Work out the finished part from the listing and answer in its coordinate system (mm). Give positions to 0.01 mm unless a question says otherwise; leave off trailing zeros. Loops run counter-clockwise (first coordinate to the right, second up) from the corner with the lowest first, then second, coordinate; pieces in that order, holes last. Notation, with made-up numbers: M 3,-31.75 L 56,-31.75 A25 cw 56,-17.75 Z; hole C -19,-5.5 d7. An arc over 180 degrees is marked long. Use a Markdown table: item, result.
```python
from build123d import *

# Parameters (mm, degrees)
SKETCH1_R                             = 19.05
EXTRUDE1_DEPTH                        = 44.45
CHAMFER1_SIZE                         = 0.762
F_3_4_0_75_DIAMETER_HOLE1_D           = 19.05
F_3_4_0_75_DIAMETER_HOLE1_DEPTH       = 36.068
F_3_4_0_75_DIAMETER_HOLE1_CSINK_D     = 20.32
F_3_4_0_75_DIAMETER_HOLE1_CSINK_ANGLE = 90
CHAMFER2_SIZE                         = 0.254


with BuildPart() as part:
    # Sketch1 → Extrude1 (new body)
    with BuildSketch(Plane(origin=(0, 0, 0), x_dir=(1, 0, 0), z_dir=(0, 1, 0))):
        with Locations(Location((0, 0, 0), (0, 0, 270))):  # turned: the seam where the file's is
            Circle(SKETCH1_R)
    extrude(amount=EXTRUDE1_DEPTH)

    # Sketch2 → 3/8 (0.375) Diameter Hole1 (revolve, cut)
    with BuildSketch(Plane(origin=(0, 44.45, 0), x_dir=(0, 0, 1), z_dir=(1, 0, 0))):
        Polygon((0, 0), (0, 44.45), (5.4102, 44.45), (4.7752, 43.815), (4.7752, 0), align=None)
    revolve(axis=Axis((0, 50.8, 0), (0, -1, 0)), mode=Mode.SUBTRACT)

    # Chamfer1
    chamfer1_edges = [part.edges().sort_by_distance(p)[0] for p in [
        (0, 0, -19.05),
        (0, 44.45, -19.05),
    ]]
    chamfer(chamfer1_edges, length=CHAMFER1_SIZE)

    # 3/4 (0.75) Diameter Hole1
    with Locations(Plane(origin=(0, 44.45, 0), x_dir=(-1, 0, 0), z_dir=(0, 1, 0))):
        with Locations((0, 0)):
            CounterSinkHole(F_3_4_0_75_DIAMETER_HOLE1_D / 2, F_3_4_0_75_DIAMETER_HOLE1_CSINK_D / 2, depth=F_3_4_0_75_DIAMETER_HOLE1_DEPTH, counter_sink_angle=F_3_4_0_75_DIAMETER_HOLE1_CSINK_ANGLE)

    # Chamfer2
    chamfer2_edges = [part.edges().sort_by_distance(p)[0] for p in [
        (-9.525, 8.382, 0),
    ]]
    chamfer(chamfer2_edges, length=CHAMFER2_SIZE)


solid = part.part
```
(1) A cutting plane is placed at B-B (x = 0). Write down the section's boundary in (y, z) (3 decimals), and give its area (3 significant figures).
Entries:
| item | result |
|---|---|
| outline | M 0,-18.288 L 0.762,-19.05 L 43.688,-19.05 L 44.45,-18.288 L 44.45,-10.16 L 43.815,-9.525 L 8.636,-9.525 L 8.382,-9.271 L 8.382,-4.775 L 0.635,-4.775 L 0,-5.41 Z; M 0,5.41 L 0.635,4.775 L 8.382,4.775 L 8.382,9.271 L 8.636,9.525 L 43.815,9.525 L 44.45,10.16 L 44.45,18.288 L 43.688,19.05 L 0.762,19.05 L 0,18.288 Z |
| area | 924 mm² |
(2) A cutting plane is placed at C-C (y = 37). Write down the section's boundary in (x, z) (3 decimals).
Entries:
| item | result |
|---|---|
| outline | C 0,0 d38.1; hole C 0,0 d19.05 |
(3) The mould has two halves that part along Z. Classify faces 1 (the flat face through (4, 8.382, -4)), 2 (the cylindrical face through (-11.59, 21.92, -15.12)), 3 (the cylindrical face through (-7.559, 25.979, -5.796)), 4 (the flat face through (-8, 44.45, 8)): released by +Z, released by -Z, zero draft, split by the parting line, or undercut.
Entries:
| item | result |
|---|---|
| face 1 | undercut |
| face 2 | split by the parting line |
| face 3 | undercut |
| face 4 | zero draft |
(4) A cutting plane is placed at A-A (z = 0). Write down the section's boundary in (x, y) (3 decimals), and give its area (3 significant figures).
Entries:
| item | result |
|---|---|
| outline | M -19.05,0.762 L -18.288,0 L -5.41,0 L -4.775,0.635 L -4.775,8.382 L -9.271,8.382 L -9.525,8.636 L -9.525,43.815 L -10.16,44.45 L -18.288,44.45 L -19.05,43.688 Z; M 4.775,0.635 L 5.41,0 L 18.288,0 L 19.05,0.762 L 19.05,43.688 L 18.288,44.45 L 10.16,44.45 L 9.525,43.815 L 9.525,8.636 L 9.271,8.382 L 4.775,8.382 Z |
| area | 924 mm² |
(5) Given P1, Ø2, axis at y = 34, z = 6.5, coming from the +X side; P2, Ø5, axis at y = 19.5, z = -6.5, coming from the +X side; P3, Ø2, axis at y = 19.5, z = 15, coming from the +X side, each flat-ended and moving along its own axis, determine where each tip first touches the part or whether it passes through.
Entries:
| item | result |
|---|---|
| P1 | stops at x = 18.24 |
| P2 | stops at x = 18.63 |
| P3 | stops at x = 12.92 |
(6) Consider probe 1 along X at (y, z) = (6, 0); probe 2 along X at (y, z) = (36, 0) (3 decimals); probe 3 along X at (y, z) = (26.5, -16.5). Determine where each line is inside the solid, lowest interval first. Write a range as [from, to].
Entries:
| item | result |
|---|---|
| probe 1 | x = [-19.05, -4.78], [4.78, 19.05] |
| probe 2 | x = [-19.05, -9.525], [9.525, 19.05] |
| probe 3 | x = [-9.52, 9.52] |
